Can you work these out from the model? Positions are in its coordinate system, mm. A direction names the side the tool comes from. Give positions to 0.01 mm unless a question says otherwise; leave off trailing zeros. Order: outer loops, then holes, each group sorted by start corner. A loop starts at its lowest first (then second) coordinate and runs counter-clockwise, first axis right, second up. Notation, with made-up numbers: (86.25, -6.5) - (118.25, -6.5) arc R16 cw to (118.25, 3.5) - close; hole circle Ø6 at (61, 7.5). An arc over 180 degrees is marked (long way). One line per question, with ' | ' between items.
```python
from build123d import *

# Parameters (mm, degrees)
SKETCH1_R           = 31
SKETCH1_R_2         = 4.5
SKETCH1_R_3         = 0.8
SKETCH1_R_4         = 1.55
BOSS_EXTRUDE2_DEPTH = 6
SKETCH5_R           = 8.2
CUT_EXTRUDE3_DEPTH  = 3
SKETCH6_R           = 3.5
CUT_EXTRUDE4_DEPTH  = 4


with BuildPart() as part:
    # Sketch1 → Boss-Extrude2 (new body)
    with BuildSketch(Plane.XY):
        Circle(SKETCH1_R)
        Circle(SKETCH1_R_2, mode=Mode.SUBTRACT)
        with Locations((8.980256121, 8.980256121)):
            Circle(SKETCH1_R_3, mode=Mode.SUBTRACT)
        with Locations((8.980256121, -8.980256121)):
            Circle(SKETCH1_R_3, mode=Mode.SUBTRACT)
        with Locations((-8.980256121, -8.980256121)):
            Circle(SKETCH1_R_3, mode=Mode.SUBTRACT)
        with Locations((-8.980256121, 8.980256121)):
            Circle(SKETCH1_R_3, mode=Mode.SUBTRACT)
        with Locations((-27, 0)):
            Circle(SKETCH1_R_4, mode=Mode.SUBTRACT)
        with Locations((-19.091883092, 19.091883092)):
            Circle(SKETCH1_R_4, mode=Mode.SUBTRACT)
        with Locations((0, 27)):
            Circle(SKETCH1_R_4, mode=Mode.SUBTRACT)
        with Locations((19.091883092, 19.091883092)):
            Circle(SKETCH1_R_4, mode=Mode.SUBTRACT)
        with Locations((27, 0)):
            Circle(SKETCH1_R_4, mode=Mode.SUBTRACT)
        with Locations((19.091883092, -19.091883092)):
            Circle(SKETCH1_R_4, mode=Mode.SUBTRACT)
        with Locations((0, -27)):
            Circle(SKETCH1_R_4, mode=Mode.SUBTRACT)
        with Locations((-19.091883092, -19.091883092)):
            Circle(SKETCH1_R_4, mode=Mode.SUBTRACT)
    extrude(amount=BOSS_EXTRUDE2_DEPTH)

    # Sketch5 → Cut-Extrude3 (cut)
    with BuildSketch(Plane(origin=(0, 0, 0), x_dir=(-1, 0, 0), z_dir=(0, 0, -1))):
        Circle(SKETCH5_R)
    extrude(amount=-CUT_EXTRUDE3_DEPTH, mode=Mode.SUBTRACT)

    # Sketch6 → Cut-Extrude4 (cut)
    with BuildSketch(Plane.XY.offset(6)):
        with Locations((0, 27)):
            Circle(SKETCH6_R)
        with Locations((19.091883092, 19.091883092)):
            Circle(SKETCH6_R)
        with Locations((27, 0)):
            Circle(SKETCH6_R)
        with Locations((19.091883092, -19.091883092)):
            Circle(SKETCH6_R)
        with Locations((0, -27)):
            Circle(SKETCH6_R)
        with Locations((-19.091883092, -19.091883092)):
            Circle(SKETCH6_R)
        with Locations((-27, 0)):
            Circle(SKETCH6_R)
        with Locations((-19.091883092, 19.091883092)):
            Circle(SKETCH6_R)
    extrude(amount=-CUT_EXTRUDE4_DEPTH, mode=Mode.SUBTRACT)


solid = part.part
```
(1) On a 3-axis mill with a long thin cutter (end or side, diameter ignored), from which of +Z, -Z, +X, -X, +Y, -Y can I reach the whole of each face in a straight line? I mean faces 4 (the face through (-26, -2, 2)), 5 (the face through (-9.615, -9.467, 2.958)). Say none if no direction works.
Answer below:
face 4: +Z | face 5: +Z, -Z
(2) Imagine slicing it at D-D (z = 5.1). Count the separate pieces of the cut face and the enclosed holes in it, and give its area (3 significant figures).
Answer below:
separate pieces: 1 | enclosed holes: 13 | area: 2,640 mm^2
(3) Will these pins go through, and if not, where does the flat tip stop? pin 1 (8 mm diameter, centred on x = 19.09, y = -19.09, fed in from +Z); pin 2 (15 mm diameter, centred on x = 0, y = 0, fed in from -Z); pin 3 (1.5 mm diameter, centred on y = -11.5, z = 3.5, fed in from -X).
Answer below:
pin 1: z = 6 | pin 2: z = 3 | pin 3: x = -29.08
(4) Imagine slicing it at A-A (x = 0). List the corners of the cut face in (y, z) for me.
Answer below:
outline: (-31, 0) - (-28.55, 0) - (-28.55, 2) - (-30.5, 2) - (-30.5, 6) - (-31, 6) - close; (-25.45, 0) - (-8.2, 0) - (-8.2, 3) - (-4.5, 3) - (-4.5, 6) - (-23.5, 6) - (-23.5, 2) - (-25.45, 2) - close; (4.5, 3) - (8.2, 3) - (8.2, 0) - (25.45, 0) - (25.45, 2) - (23.5, 2) - (23.5, 6) - (4.5, 6) - close; (28.55, 0) - (31, 0) - (31, 6) - (30.5, 6) - (30.5, 2) - (28.55, 2) - close
(5) If I drill on line 1 (Y direction, x = 0, z = 2.35); line 2 (Y direction, x = -18, z = 0.3); line 3 (Y direction, x = 19.5, z = 3), over which ranges is the centre line in solid material (lowest first)?
Answer below:
line 1: -31 to -30.5, -23.5 to -8.2, 8.2 to 23.5, 30.5 to 31 | line 2: -25.24 to -20.19, -17.99 to 17.99, 20.19 to 25.24 | line 3: -24.1 to -22.57, -15.62 to 15.62, 22.57 to 24.1
(6) Imagine slicing it at C-C (x = -27). List the corners of the cut face in (y, z) for me, and give its area (3 significant figures).
Answer below:
outline: (-15.23, 0) - (-1.55, 0) - (-1.55, 2) - (-3.5, 2) - (-3.5, 6) - (-15.23, 6) - close; (1.55, 0) - (15.23, 0) - (15.23, 6) - (3.5, 6) - (3.5, 2) - (1.55, 2) - close | area: 149 mm^2
(7) If we mould it in two halves opening along X, with no side actions, what happens to faces 1 (the face through (-4.036, 30.736, 2.958)), 2 (the face through (0, -6, 6)), 3 (the face through (21, -20, 2))? For each: released by +X, released by -X, zero draft, split by the parting line, or undercut.
Answer below:
face 1: split by the parting line | face 2: zero draft | face 3: undercut
